Model file for the job. Use its own axes, mm. A direction names the side the tool comes from. Give positions to 0.01 mm unless a question says otherwise; leave off trailing zeros. Write each loop counter-clockwise with the first axis right and the second up, starting at its lowest first coordinate (ties: lowest second). Pieces come first, ordered by that corner, then holes.
```python
from build123d import *

# Parameters (mm, degrees)
ESQUISSE1_W                                       = 45.3
ESQUISSE1_H                                       = 40
BOSS_EXTRU_1_DEPTH                                = 7
CHAMBRAGE_POUR_VIS_SIX_PANS_CREUX_M42_D           = 4
CHAMBRAGE_POUR_VIS_SIX_PANS_CREUX_M42_CBORE_D     = 6
CHAMBRAGE_POUR_VIS_SIX_PANS_CREUX_M42_CBORE_DEPTH = 3
ESQUISSE8_R                                       = 8.5
ENL_V_MAT_EXTRU_1_DEPTH                           = 7
CHAMBRAGE_POUR_VIS_SIX_PANS_CREUX_M43_D           = 4
CHAMBRAGE_POUR_VIS_SIX_PANS_CREUX_M43_CBORE_D     = 6
CHAMBRAGE_POUR_VIS_SIX_PANS_CREUX_M43_CBORE_DEPTH = 3


with BuildPart() as part:
    # Esquisse1 → Boss.-Extru.1 (new body)
    with BuildSketch(Plane.XY):
        with Locations((3.477385892, 0.545435685)):
            Rectangle(ESQUISSE1_W, ESQUISSE1_H)
    extrude(amount=-BOSS_EXTRU_1_DEPTH)

    # Chambrage pour vis à six pans creux M42 (through all)
    with Locations(Plane(origin=(0, 0, -7), x_dir=(-1, 0, 0), z_dir=(0, 0, -1))):
        with Locations((-22.627385892, 17.045435685), (15.672614108, 17.045435685), (15.672614108, -15.954564315), (-22.627385892, -15.954564315)):
            CounterBoreHole(CHAMBRAGE_POUR_VIS_SIX_PANS_CREUX_M42_D / 2, CHAMBRAGE_POUR_VIS_SIX_PANS_CREUX_M42_CBORE_D / 2, CHAMBRAGE_POUR_VIS_SIX_PANS_CREUX_M42_CBORE_DEPTH)

    # Esquisse8 → Enlèv. mat.-Extru.1 (cut)
    with BuildSketch(Plane(origin=(0, 0, -7), x_dir=(-1, 0, 0), z_dir=(0, 0, -1))):
        with Locations((-5.682958625, 5.866379902)):
            Circle(ESQUISSE8_R)
    extrude(amount=-ENL_V_MAT_EXTRU_1_DEPTH, mode=Mode.SUBTRACT)

    # Chambrage pour vis à six pans creux M43 (through all)
    with Locations(Plane(origin=(0, 0, -7), x_dir=(-1, 0, 0), z_dir=(0, 0, -1))):
        with Locations((-5.627385892, -13.954564315), (-18.127385892, -5.454564315), (10.172614108, 6.545435685)):
            CounterBoreHole(CHAMBRAGE_POUR_VIS_SIX_PANS_CREUX_M43_D / 2, CHAMBRAGE_POUR_VIS_SIX_PANS_CREUX_M43_CBORE_D / 2, CHAMBRAGE_POUR_VIS_SIX_PANS_CREUX_M43_CBORE_DEPTH)


solid = part.part
```
1. Slice it at C-C, the plane y = 7.5. Write the cut outline in (x, z).
Calculated:
outline: (-19.17, -7) - (-13.02, -7) - (-13.02, -4) - (-11.93, -4) - (-11.93, 0) - (-19.17, 0) - close; (-8.42, -4) - (-7.33, -4) - (-7.33, -7) - (-2.66, -7) - (-2.66, 0) - (-8.42, 0) - close; (14.02, -7) - (26.13, -7) - (26.13, 0) - (14.02, 0) - close
2. Pin check, flat tips, straight feed: P1, Ø2.5, axis at x = -10.17, y = 6.55, coming from the +Z side; P2, Ø3, axis at x = 22.5, y = 16.5, coming from the -Z side. Stop position of each tip, or through.
Calculated:
P1: passes through
P2: stops at z = -4
3. Slice it at B-B, the plane x = -9.5. Write the cut outline in (y, z).
Calculated:
outline: (-19.45, -7) - (3.62, -7) - (3.62, -4) - (4.66, -4) - (4.66, 0) - (-19.45, 0) - close; (8.43, -4) - (9.47, -4) - (9.47, -7) - (20.55, -7) - (20.55, 0) - (8.43, 0) - close
4. Which spindle directions (+Z, -Z, +X, -X, +Y, -Y) get a long thin tool onto all of the face, cutting with end or side? Do faces 1 (the flat face through (8, -14, -4)), 2 (the cylindrical face through (5.37, -11.97, -1.97)). Say none if no direction does.
Calculated:
face 1: -Z
face 2: +Z, -Z
5. Slice it at D-D, the plane z = -6.5. State how many separate pieces and enclosed holes the cut face has, and give its area (3 significant figures).
Calculated:
separate pieces: 1
enclosed holes: 8
area: 1,390 mm2
6. Pull direction X, two halves, no side cores. Call faces 3 (the flat face through (16, -6, -4)), 4 (the flat face through (-8, 7, -4)), 5 (the flat face through (-19.173, 0, -3)), 6 (the flat face through (-2, 1, -7)): +X half, -X half, draft (parallel to the pull), parting line (faces both ways), or undercut.
Calculated:
face 3: undercut
face 4: undercut
face 5: -X half
face 6: draft
7. Slice it at A-A, the plane x = 6. Write the cut outline in (y, z).
Calculated:
outline: (-19.45, -7) - (-16.93, -7) - (-16.93, -4) - (-15.92, -4) - (-15.92, 0) - (-19.45, 0) - close; (-11.99, -4) - (-10.98, -4) - (-10.98, -7) - (-2.63, -7) - (-2.63, 0) - (-11.99, 0) - close; (14.36, -7) - (20.55, -7) - (20.55, 0) - (14.36, 0) - close
8. Probe probe 1 along Y at (x, z) = (23.5, -1.5); probe 2 along Y at (x, z) = (-16.5, -3); probe 3 along Z at (x, y) = (4, -16). List the from-to ranges inside material, lowest first.
Calculated:
probe 1: y = -19.45 to -17.75, -14.15 to 15.25, 18.85 to 20.55
probe 2: y = -19.45 to -17.78, -14.13 to 15.22, 18.87 to 20.55
probe 3: z = -4 to 0
